Part model, mm, in its own coordinate system. Give positions to 0.01 mm unless a question says otherwise; leave off trailing zeros. Write each loop counter-clockwise with the first axis right and the second up, starting at its lowest first coordinate (ties: lowest second). Pieces come first, ordered by that corner, then holes. Notation, with made-up numbers: (55.25, 81) - (91.25, 81) arc R11 cw to (91.25, 100) - close; hole circle Ø2 at (-1.5, 85.25). An arc over 180 degrees is marked (long way). Answer in a Markdown table with one row per item. Add a question column.
1. Drop a flat-ended pin along its axis: pin 1 Ø5 at (x, z) = (95, 17) entering from -Y. Give the stop position or say it passes through.
2. Band-saw the part on C-C on x = 83. Write the cut outline in (y, z).
3. Probe line 1 along Y through (x, z) = (43, 4); line 2 along Y through (x, z) = (61.5, 15); line 3 along X through (y, z) = (316.5, 2). List the from-to ranges inside material, lowest first.
4. Band-saw the part on B-B on z = 10.5. Write the cut outline in (x, y).
5. Band-saw the part on D-D on y = 299. Write the cut outline in (x, z), plus the area to 3 significant figures.
6. Band-saw the part on A-A on x = 55. Write the cut outline in (y, z).
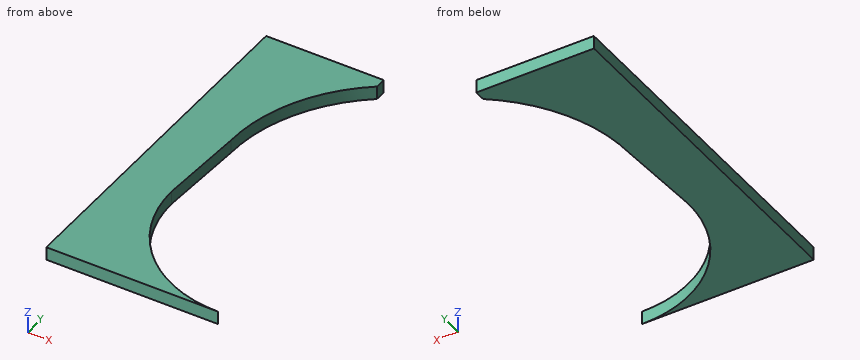
Autodesk Inventor part; units mm, degrees
ref_plane "YZ Plane" through (0, 0, 0) normal (1, 0, 0) x (0, 1, 0)
ref_plane "XZ Plane" through (0, 0, 0) normal (0, 1, 0) x (-1, 0, 0)
ref_plane "XY Plane" through (0, 0, 0) normal (0, 0, 1) x (1, 0, 0)
sketch "Sketch1" plane through (0, 0, 0) normal (0, 0, 1) x (1, 0, 0)
  line L0 (0, 0) -> (609.6, 0) construction
  line L1 (609.6, 0) -> (609.6, 209.55)
  line L2 (609.6, 209.55) -> (0, 209.55) construction
  line L3 (0, 209.55) -> (0, 0) construction
  line L4 (0, 0) -> (304.8, 0) construction
  line L5 (304.8, 0) -> (304.8, 165.1) construction
  line L6 (304.8, 165.1) -> (0, 165.1) construction
  line L7 (0, 165.1) -> (0, 0) construction
  line L8 (0, 0) -> (165.1, 0) construction
  line L9 (165.1, 0) -> (165.1, 304.8) construction
  line L10 (165.1, 304.8) -> (0, 304.8) construction
  line L11 (0, 304.8) -> (0, 0) construction
  line L12 (0, 0) -> (177.8, 0) construction
  line L13 (177.8, 0) -> (177.8, 177.8) construction
  line L14 (177.8, 177.8) -> (0, 177.8) construction
  line L15 (0, 177.8) -> (0, 0) construction
  circle A0 centre (177.8, 177.8) radius 12.7
  line L16 (177.8, 177.8) -> (165.1, 177.8)
  line L17 (177.8, 177.8) -> (177.8, 165.1)
  line L18 (177.8, 177.8) -> (168.8197, 168.8197)
  line L19 (177.8, 177.8) -> (190.5, 177.8) construction
  line L20 (168.8197, 168.8197) -> (52.0764, 52.0764) construction
  line L21 (168.8197, 168.8197) -> (333.9197, 168.8197) construction
  line L22 (177.8, 165.1) -> (177.8, 0) construction
  line L23 (165.1, 177.8) -> (0, 177.8) construction
  arc A1 (0, 177.8) -> (177.8, 0) centre (177.8, 177.8) ccw
  line L24 (177.8, 177.8) -> (355.6, 177.8) construction
  line L25 (355.6, 177.8) -> (355.6, 193.675)
  line L26 (355.6, 193.675) -> (177.8, 193.675) construction
  line L27 (177.8, 193.675) -> (177.8, 177.8) construction
  circle A2 centre (355.6, 193.675) radius 12.7
  line L28 (355.6, 193.675) -> (482.6, 193.675) construction
  line L29 (482.6, 209.55) -> (355.6, 209.55) construction
  line L30 (355.6, 209.55) -> (355.6, 193.675) construction
  line L31 (177.8, 0) -> (609.6, 0)
  line L32 (177.8, 165.1) -> (355.6, 180.975)
  line L33 (165.1, 177.8) -> (165.1, 304.8) construction
  line L34 (165.1, 304.8) -> (241.3, 304.8) construction
  circle A3 centre (241.3, 304.8) radius 76.2
  circle A4 centre (177.8, 228.6) radius 12.7
  line L35 (177.8, 177.8) -> (177.8, 228.6)
  line L36 (241.3, 304.8) -> (195.4417, 365.656) construction
  line L37 (241.3, 304.8) -> (317.5, 304.8) construction
  line L38 (195.4417, 365.656) -> (354.1917, 365.656) construction
  line L39 (195.4417, 365.656) -> (99.9036, 492.4394) construction
  line L40 (195.4417, 365.656) -> (354.1917, 365.656) construction
  line L41 (165.1, 304.8) -> (0, 304.8) construction
  line L42 (241.3, 304.8) -> (169.6954, 330.8619) construction
  line L43 (241.3, 304.8) -> (317.5, 304.8) construction
  line L44 (169.6954, 330.8619) -> (20.5192, 385.1576) construction
  line L45 (177.8, 0) -> (408.0964, 0) construction
  line L46 (241.3, 304.8) -> (317.5, 304.8) construction
  line L47 (241.3, 304.8) -> (175.3089, 342.9) construction
  line L48 (241.3, 304.8) -> (317.5, 304.8) construction
  line L49 (175.3089, 342.9) -> (37.8273, 422.275) construction
  line L50 (190.5, 177.8) -> (393.7, 177.8) construction
  line L51 (609.6, 0) -> (-50.8, 0)
  line L52 (-50.8, 0) -> (-50.8, 508)
  line L53 (177.8, 0) -> (-50.8, 0)
  line L54 (-50.8, 492.4394) -> (-50.8, 508)
  line L55 (-50.8, 508) -> (99.9036, 508)
  line L56 (99.9036, 508) -> (99.9036, 492.4394)
  line L57 (355.6, 180.975) -> (609.6, 209.55)
  arc A5 (99.9036, 492.4394) -> (6.35, 304.8) centre (241.3, 304.8) ccw
  line L58 (0, 177.8) -> (6.35, 304.8)
  line L59 (0, 304.8) -> (0, 177.8) construction
  line L60 (6.35, 304.8) -> (0, 304.8) construction
  point P0 (165.2751, 230.7014)
  point P1 (172.7151, 216.9624)
  dimension "d16" = 25.4
  dimension "d0" = 609.6
  dimension "d1" = 209.55
  dimension "d2" = 304.8
  dimension "d3" = 165.1
  dimension "d4" = 165.1
  dimension "d5" = 304.8
  dimension "d6" = 177.8
  dimension "d7" = 177.8
  dimension "d8" = 25.4
  dimension "d9" = 12.7
  dimension "d10" = 135
  dimension "d11" = 165.1
  dimension "d12" = 135
  dimension "d13" = 165.1
  dimension "d14" = 177.8
  dimension "d15" = 15.875
  dimension "d17" = 127
  dimension "d20" = 127
  dimension "d21" = 76.2
  dimension "d22" = 152.4
  dimension "d23" = 25.4
  dimension "d24" = 50.8
  dimension "d26" = 127
  dimension "d33" = 158.75
  dimension "d34" = 127
  dimension "d35" = 160
  dimension "d36" = 158.75
  dimension "d37" = 180
  dimension "d45" = 150
  dimension "d46" = 158.75
  dimension "d47" = 180
  dimension "d72" = 660.4
  dimension "d73" = 508
  dimension "d74" = 90
  dimension "d77" = 150.7036
  dimension "d78" = 15.5606
extrude "Extrusion2" add sketch "Sketch1" along normal blind 19.05 contours A1 L51 L52 L55 L56 A5 L58
move faces "Move1" translate (-19.05, 0, 0) faces at (-50.8, 338.6667, 6.35)
Values:
| question | item | result |
|---|---|---|
| 1 | pin 1 | stops at y = 0 |
| 2 | outline | (0, 0) - (27.38, 0) - (27.38, 19.05) - (0, 19.05) - close; (478.42, 0) - (508, 0) - (508, 19.05) - (478.42, 19.05) - close |
| 3 | line 1 | y = 0 to 61.86, 430.81 to 508 |
| 3 | line 2 | y = 0 to 43.31, 456.04 to 508 |
| 3 | line 3 | x = -69.85 to 6.64 |
| 4 | outline | (-69.85, 0) - (177.8, 0) arc R177.8 cw to (0, 177.8) - (6.35, 304.8) arc R234.95 cw to (99.9, 492.44) - (99.9, 508) - (-69.85, 508) - close |
| 5 | outline | (-69.85, 0) - (6.06, 0) - (6.06, 19.05) - (-69.85, 19.05) - close |
| 5 | area | 1,450 mm² |
| 6 | outline | (0, 0) - (49.22, 0) - (49.22, 19.05) - (0, 19.05) - close; (447.96, 0) - (508, 0) - (508, 19.05) - (447.96, 19.05) - close |
